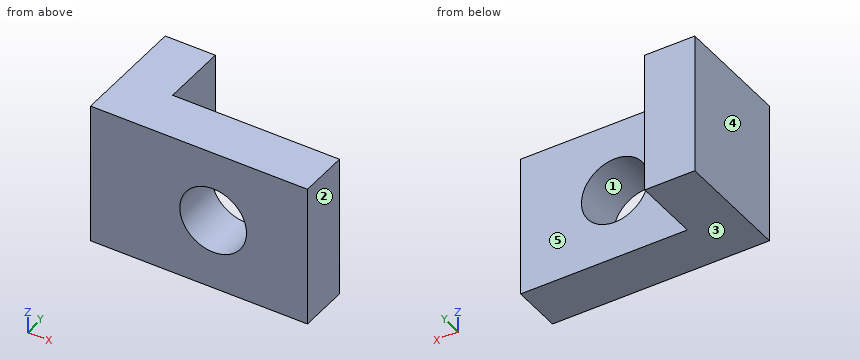
```python
from build123d import *

# Parameters (mm, degrees)
SKETCH1_W           = 13
SKETCH1_H           = 8.5
BOSS_EXTRUDE2_DEPTH = 3
SKETCH2_R           = 2
CUT_EXTRUDE1_DEPTH  = 9.325412903
SKETCH3_W           = 3
SKETCH3_H           = 8.5
BOSS_EXTRUDE3_DEPTH = 4


with BuildPart() as part:
    # Sketch1 → Boss-Extrude2 (new body)
    with BuildSketch(Plane(origin=(0, 0, 0), x_dir=(1, 0, 0), z_dir=(0, 1, 0))):
        Rectangle(SKETCH1_W, SKETCH1_H)
    extrude(amount=BOSS_EXTRUDE2_DEPTH)

    # Sketch2 → Cut-Extrude1 (cut, through all)
    with BuildSketch(Plane(origin=(0, 0, 0), x_dir=(1, 0, 0), z_dir=(0, 1, 0))):
        with Locations(Location((0.85, 0, 0), (0, 0, 270))):
            Circle(SKETCH2_R)
    extrude(amount=CUT_EXTRUDE1_DEPTH, mode=Mode.SUBTRACT)

    # Sketch3 → Boss-Extrude3 (add)
    with BuildSketch(Plane(origin=(0, 3, 0), x_dir=(1, 0, 0), z_dir=(0, 1, 0))):
        with Locations((-5, 0)):
            Rectangle(SKETCH3_W, SKETCH3_H)
    extrude(amount=BOSS_EXTRUDE3_DEPTH)


solid = part.part
```
Could you check a few things on this model? Use its own coordinates, in mm. Face numbers are marked on the shaded views. A direction names the side the tool comes from. Coordinates: 2 decimals unless noted, no trailing zeros. Write each loop counter-clockwise with the first axis right and the second up, starting at its lowest first coordinate (ties: lowest second). Pieces come first, ordered by that corner, then holes. Notation, with made-up numbers: (44.25, 59) - (83.25, 59) arc R21 cw to (83.25, 90) - close; hole circle Ø4 at (36, 14.5). An arc over 180 degrees is marked (long way). Use a Markdown table: item, result.
Q1. Please list where these lines run through material, in increasing order: L1, parallel to Z at x = 0.85, y = 0.9; L2, parallel to X at y = 1.1, z = 0; L3, parallel to Y at x = -1.25, z = -2.5.
Geometry check:
| item | result |
|---|---|
| L1 | z = -4.25 to -2, 2 to 4.25 |
| L2 | x = -6.5 to -1.15, 2.85 to 6.5 |
| L3 | y = 0 to 3 |
Q2. Imagine slicing it at B-B (x = 0.85). List the corners of the cut face in (y, z) for me, and give its area (3 significant figures).
Geometry check:
| item | result |
|---|---|
| outline | (0, -4.25) - (3, -4.25) - (3, -2) - (0, -2) - close; (0, 2) - (3, 2) - (3, 4.25) - (0, 4.25) - close |
| area | 13.5 mm2 |
Q3. Imagine slicing it at C-C (y = 0.5). List the corners of the cut face in (x, z) for me.
Geometry check:
| item | result |
|---|---|
| outline | (-6.5, -4.25) - (6.5, -4.25) - (6.5, 4.25) - (-6.5, 4.25) - close; hole circle Ø4 at (0.85, 0) |
Q4. Imagine slicing it at D-D (z = 3). List the corners of the cut face in (x, y) for me.
Geometry check:
| item | result |
|---|---|
| outline | (-6.5, 0) - (6.5, 0) - (6.5, 3) - (-3.5, 3) - (-3.5, 7) - (-6.5, 7) - close |
Q5. Thinking about a two-plate mould opening in Z: for the marked faces 1, 2 and 3, which applies, +Z half, -Z half, draft (parallel to the pull), parting line (faces both ways), or undercut?
Geometry check:
| item | result |
|---|---|
| face 1 | undercut |
| face 2 | draft |
| face 3 | -Z half |
Q6. Imagine slicing it at A-A (z = 0). List the corners of the cut face in (x, y) for me, and give its area (3 significant figures).
Geometry check:
| item | result |
|---|---|
| outline | (-6.5, 0) - (-1.15, 0) - (-1.15, 3) - (-3.5, 3) - (-3.5, 7) - (-6.5, 7) - close; (2.85, 0) - (6.5, 0) - (6.5, 3) - (2.85, 3) - close |
| area | 39.0 mm2 |
Q7. I'm going to push flat-ended pins straight in: pin 1 Ø3.5 at (x, z) = (0.85, 0) entering from +Y (3 decimals); pin 2 Ø2 at (y, z) = (5, 1.5) entering from +X; pin 3 Ø3 at (x, z) = (-1.5, 3.5) entering from -Y; pin 4 Ø2.5 at (x, z) = (2.5, -0.5) entering from +Y. Where does each tip first touch, or does it pass through?
Geometry check:
| item | result |
|---|---|
| pin 1 | passes through |
| pin 2 | stops at x = -3.5 |
| pin 3 | stops at y = 0 |
| pin 4 | stops at y = 3 |
Q8. Which directions (+Z, -Z, +X, -X, +Y, -Y) give clear straight access to the entire face, cutting with the end or side of a thin tool? Please do the marked faces 4 and 5.
Geometry check:
| item | result |
|---|---|
| face 4 | +Z, -Z, -X, +Y, -Y |
| face 5 | +Z, -Z, +X, +Y |
